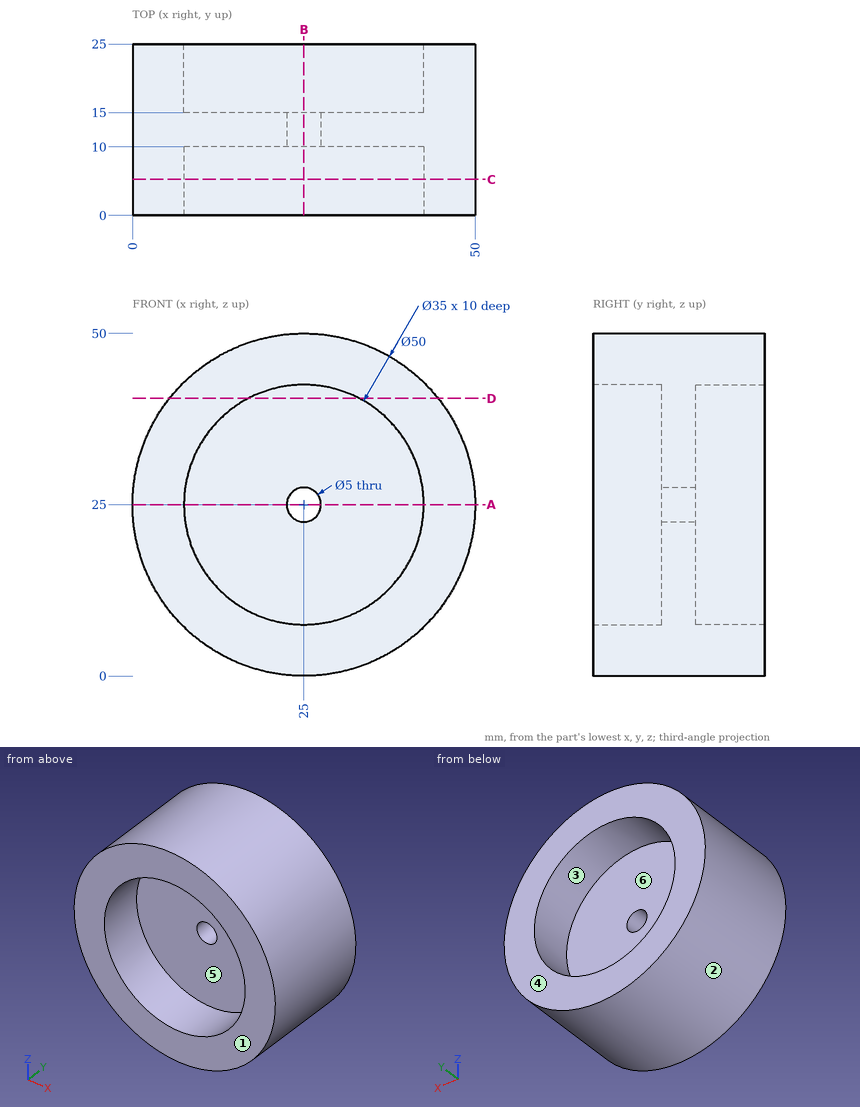
Part print with two shaded views. Sizes in mm from the minimum x, y, z corner. A direction names the side the tool comes from. Round coordinates to 2 decimals unless told otherwise and drop trailing zeros. Loops run counter-clockwise (first coordinate to the right, second up) from the corner with the lowest first, then second, coordinate; pieces in that order, holes last. Notation, with made-up numbers: M -38,12.25 L -27,12.25 A20 cw -27,43.25 Z; hole C 76,21.25 d6. An arc over 180 degrees is marked long. Put each result on its own line as item: value. Start each with the question number.
Item 1: Drop flat-ended pins along their axis: P1, Ø2, axis at x = 35, y = 15, coming from the -Z side; P2, Ø1, axis at x = 30, y = 11.5, coming from the -Z side; P3, Ø12, axis at x = 36.5, y = 21.5, coming from the -Z side. Give the stop position or say it passes through.
Item 2: Cut at A-A (z = 25). List the corners of the cut face in (x, y), then the cut area to 3 significant figures.
Item 3: Cut at B-B (x = 25). List the corners of the cut face in (y, z).
Item 4: Drill centre lines: line 1 along X through (y, z) = (13.1, 25); line 2 along X through (y, z) = (18, 25); line 3 along Y through (x, z) = (31.5, 9). Where is each one in solid material? Low to high.
Item 5: Mould opens along X. For the marked faces 1, 2 and 3 say: released by +X, released by -X, zero draft, split by the parting line, or undercut.
Item 6: 3-axis set-ups, long thin cutter, end or side, ignore diameter. For the marked faces 4, 5 and 6: which of +Z, -Z, +X, -X, +Y, -Y reach the whole face in a straight line?
Item 7: Cut at C-C (y = 5.25). List the corners of the cut face in (x, z), then the cut area to 3 significant figures.
Item 8: Cut at D-D (z = 40.5). List the corners of the cut face in (x, y).
Answer block:
1. P1: z = 1.68
1. P2: z = 0.41
1. P3: z = 0.61
2. outline: M 0,0 L 7.5,0 L 7.5,10 L 22.5,10 L 22.5,15 L 7.5,15 L 7.5,25 L 0,25 Z; M 27.5,10 L 42.5,10 L 42.5,0 L 50,0 L 50,25 L 42.5,25 L 42.5,15 L 27.5,15 Z
2. area: 525 mm2
3. outline: M 0,0 L 25,0 L 25,7.5 L 15,7.5 L 15,22.5 L 10,22.5 L 10,7.5 L 0,7.5 Z; M 0,42.5 L 10,42.5 L 10,27.5 L 15,27.5 L 15,42.5 L 25,42.5 L 25,50 L 0,50 Z
4. line 1: 0 to 22.5, 27.5 to 50
4. line 2: 0 to 7.5, 42.5 to 50
4. line 3: 10 to 15
5. face 1: zero draft
5. face 2: split by the parting line
5. face 3: undercut
6. face 4: +Z, -Z, +X, -X, +Y
6. face 5: -Y
6. face 6: +Y
7. outline: C 25,25 d50; hole C 25,25 d35
7. area: 1,000 mm2
8. outline: M 5.38,0 L 16.88,0 L 16.88,10 L 33.12,10 L 33.12,0 L 44.62,0 L 44.62,25 L 33.12,25 L 33.12,15 L 16.88,15 L 16.88,25 L 5.38,25 Z
